Part print with two shaded views. Sizes in mm from the minimum x, y, z corner. Coordinates: 2 decimals unless noted, no trailing zeros. Write each loop counter-clockwise with the first axis right and the second up, starting at its lowest first coordinate (ties: lowest second). Pieces come first, ordered by that corner, then holes.
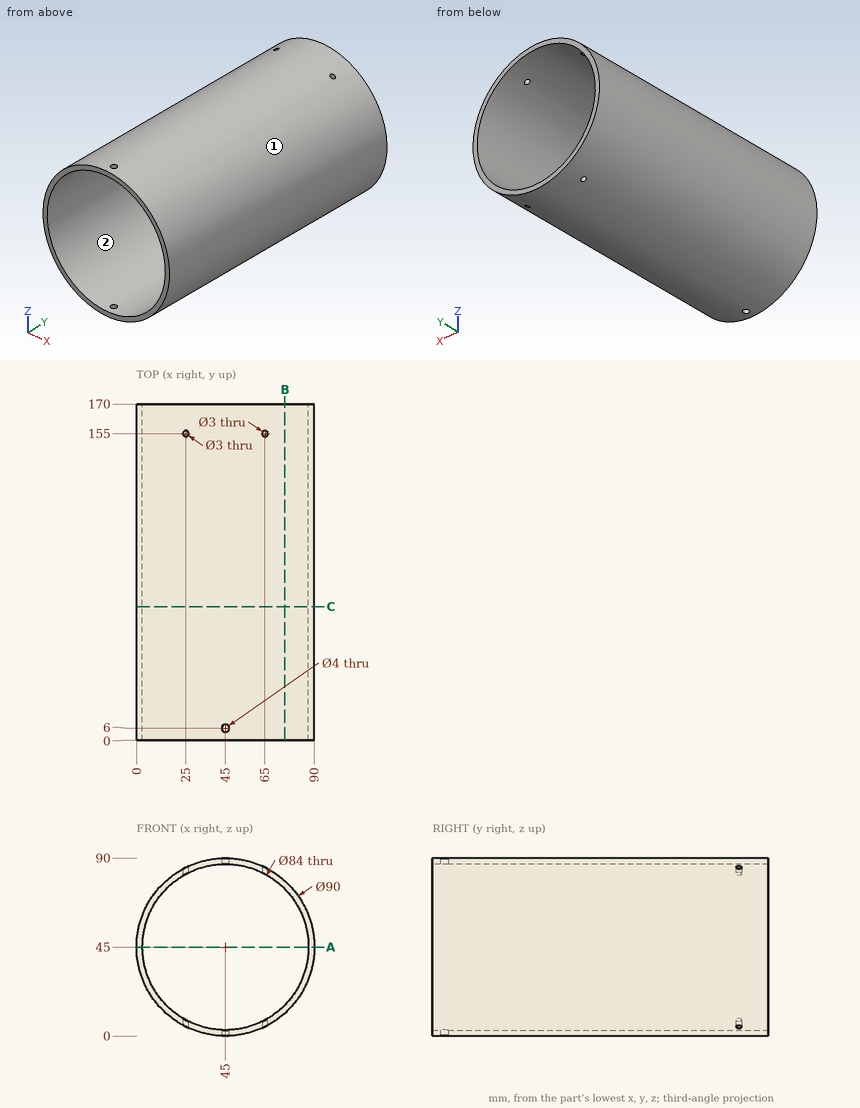
(1) Two-plate mould, pull along X, no slides. Class the marked faces 1 and 2: pulls with the +X half, pulls with the -X half, needs draft (parallel to the pull), parting line crosses it, or undercut.
(2) Slice it at C-C, the plane y = 67.5. List the corners of the cut face in (x, z).
(3) Probe L1, parallel to Y at x = 25, z = 82; L2, parallel to X at y = 57, z = 45; L3, parallel to X at y = 44, z = 69. List the from-to ranges inside material, lowest first.
(4) Slice it at A-A, the plane z = 45. List the corners of the cut face in (x, y), and give its area (3 significant figures).
(5) Slice it at B-B, the plane x = 75. List the corners of the cut face in (y, z).
(6) Flat gauge pins, fed straight in: P1, Ø2, axis at x = 23, y = 132.5, coming from the +Z side; P2, Ø4, axis at x = 65, y = 155, coming from the +Z side; P3, Ø3.5, axis at x = 25, y = 155, coming from the -Z side; P4, Ø6.5, axis at x = 45, y = 6, coming from the -Z side. Where does each tip first touch, or does it go through?
Results:
1. face 1: parting line crosses it
1. face 2: undercut
2. outline: circle Ø90 at (45, 45); hole circle Ø84 at (45, 45)
3. L1: y = 0 to 153.5, 156.5 to 170
3. L2: x = 0 to 3, 87 to 90
3. L3: x = 6.93 to 10.53, 79.47 to 83.07
4. outline: (0, 0) - (3, 0) - (3, 170) - (0, 170) - close; (87, 0) - (90, 0) - (90, 170) - (87, 170) - close
4. area: 1,020 mm2
5. outline: (0, 11.46) - (170, 11.46) - (170, 15.61) - (0, 15.61) - close; (0, 74.39) - (170, 74.39) - (170, 78.54) - (0, 78.54) - close
6. P1: stops at z = 84.8
6. P2: stops at z = 86.24
6. P3: stops at z = 3.87
6. P4: stops at z = 0
